Work out the finished part from the listing and answer in its coordinate system (mm). Face numbers are marked on the shaded views. A direction names the side the tool comes from. Round coordinates to 2 decimals unless told otherwise and drop trailing zeros. Order: outer loops, then holes, each group sorted by start corner. A loop starts at its lowest first (then second) coordinate and runs counter-clockwise, first axis right, second up. Notation, with made-up numbers: (13.25, 60) -> (41.25, 60) arc R27 cw to (41.25, 94) -> close; hole circle Ø9 at (3.25, 20). An arc over 180 degrees is marked (long way). Use a Markdown table: item, result. Add a question column.
Item 1: A cutting plane is placed at B-B, the plane z = 44. Determine the outline of the cut face in (x, y), plus the area to 3 significant figures.
Item 2: Flat-ended cylindrical pins translate along their axes: P1, Ø1, axis at y = -2.5, z = 32, coming from the -X side; P2, Ø8, axis at y = -5, z = 10, coming from the +X side; P3, Ø5, axis at y = 2, z = 54.5, coming from the -X side. Find the tip coordinate at first contact, or state that the pin passes through.
Item 3: A cutting plane is placed at A-A, the plane z = 13. Determine the outline of the cut face in (x, y), plus the area to 3 significant figures.
Item 4: Find the intervals of material crossed by L1, parallel to Y at x = 40, z = 55.75; L2, parallel to Z at x = 35, y = 5.5; L3, parallel to X at y = -1, z = 54, in increasing order. Write a range as [from, to].
Item 5: A cutting plane is placed at C-C, the plane x = -48.5. Determine the outline of the cut face in (y, z).
Item 6: A cutting plane is placed at D-D, the plane y = -12. Determine the outline of the cut face in (x, z), plus the area to 3 significant figures.
Item 7: For a pull along Z with two mould halves and no side action, classify the marked faces 1, 2, 3 and 4 as +Z half, -Z half, draft (parallel to the pull), parting line (faces both ways), or undercut.
Item 8: A tool of negligible diameter and unlimited length cuts with its end or side. For the marked faces 5, 6, 7 and 8, from which of +Z, -Z, +X, -X, +Y, -Y can it reach the whole face along a straight path? Write none if from no direction.
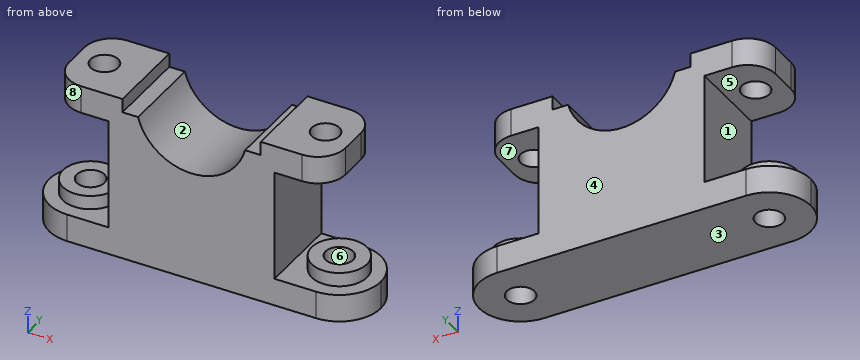
from build123d import *

# Parameters (mm, degrees)
F1_DEPTH         = 15
F2_R             = 10
F3_R             = 14.99999
F4_R             = 5
F5_DEPTH         = 10
F6_R             = 10
F7_DEPTH         = 5
F8_R             = 10
F9_DEPTH         = 5
F12_D            = 10
F12_DEPTH        = 15.001
F12_ON_F11_D     = 10
F12_ON_F11_DEPTH = 15.001


# Not quite as in the source:
# - a fillet or chamfer is up to 0.001 mm smaller than in the source, because OpenCascade refuses the exact size


with BuildPart() as f1:
    # F0 (on Front) → F1 (new body, symmetric)
    with BuildSketch(Plane.XZ):
        with BuildLine():
            Line((-60, 10), (-60, 0))
            Line((-60, 0), (60, 0))
            Line((60, 0), (60, 10))
            Line((60, 10), (30, 10))
            Line((30, 10), (30, 50))
            Line((30, 50), (50, 50))
            Line((50, 50), (50, 60))
            Line((50, 60), (25, 60))
            Line((25, 60), (25, 55))
            Line((25, 55), (19.364916731, 55))
            ThreePointArc((19.364916731, 55), (0, 40), (-19.364916731, 55))
            Line((-19.364916731, 55), (-25, 55))
            Line((-25, 55), (-25, 60))
            Line((-25, 60), (-50, 60))
            Line((-50, 60), (-50, 50))
            Line((-50, 50), (-30, 50))
            Line((-30, 50), (-30, 10))
            Line((-30, 10), (-60, 10))
        make_face()
    extrude(amount=F1_DEPTH, both=True)

    # F2
    f2_edges = [f1.edges().sort_by_distance(p)[0] for p in [
        (-50, -15, 55),
        (50, -15, 55),
        (50, 15, 55),
        (-50, 15, 55),
    ]]
    fillet(f2_edges, radius=F2_R)

    # F3 (radius 15 in the source; OpenCascade refuses exactly that, so slightly less here)
    f3_edges = [f1.edges().sort_by_distance(p)[0] for p in [
        (60, 15, 5),
        (-60, 15, 5),
        (-60, -15, 5),
        (60, -15, 5),
    ]]
    fillet(f3_edges, radius=F3_R)

    # F4 (on face) → F5 (cut, through all)
    with BuildSketch(Plane.XY.offset(60)):
        with Locations((40, 0)):
            Circle(F4_R)
        with Locations((-40, 0)):
            Circle(F4_R)
    extrude(amount=-F5_DEPTH, mode=Mode.SUBTRACT)

    # F6 (on face) → F7 (join)
    with BuildSketch(Plane.XY.offset(10)):
        with Locations((45, 0)):
            Circle(F6_R)
    extrude(amount=F7_DEPTH)

    # F8 (on face) → F9 (join)
    with BuildSketch(Plane.XY.offset(10)):
        with Locations((-45, 0)):
            Circle(F8_R)
    extrude(amount=F9_DEPTH)

    # F12 (through all, one way)
    with BuildSketch(Plane.XY.offset(15)):
        with Locations((-45, 0)):
            Circle(F12_D / 2)
    extrude(amount=-F12_DEPTH, mode=Mode.SUBTRACT)

    # F12 on F11 (through all, one way)
    with BuildSketch(Plane.XY.offset(15)):
        with Locations((45, 0)):
            Circle(F12_ON_F11_D / 2)
    extrude(amount=-F12_ON_F11_DEPTH, mode=Mode.SUBTRACT)


solid = f1.part
Reported:
| question | item | result |
|---|---|---|
| 1 | outline | (-30, -15) -> (-12, -15) -> (-12, 15) -> (-30, 15) -> close; (12, -15) -> (30, -15) -> (30, 15) -> (12, 15) -> close |
| 1 | area | 1,080 mm² |
| 2 | P1 | x = -30 |
| 2 | P2 | x = 59.97 |
| 2 | P3 | x = -50 |
| 3 | outline | circle Ø20 at (-45, 0); (-30, -15) -> (30, -15) -> (30, 15) -> (-30, 15) -> close; circle Ø20 at (45, 0); hole circle Ø10 at (-45, 0); hole circle Ø10 at (45, 0) |
| 3 | area | 2,270 mm² |
| 4 | L1 | [-15, -5], [5, 15] |
| 4 | L2 | [0, 10], [50, 60] |
| 4 | L3 | [-50, -44.9], [-35.1, -19.08], [19.08, 35.1], [44.9, 50] |
| 5 | outline | (-14.59, 0) -> (-3.57, 0) -> (-3.57, 15) -> (-9.37, 15) -> (-9.37, 10) -> (-14.59, 10) -> close; (-10.27, 50) -> (10.27, 50) -> (10.27, 60) -> (-10.27, 60) -> close; (3.57, 0) -> (14.59, 0) -> (14.59, 10) -> (9.37, 10) -> (9.37, 15) -> (3.57, 15) -> close |
| 6 | outline | (-54, 0) -> (54, 0) -> (54, 10) -> (30, 10) -> (30, 50) -> (47.14, 50) -> (47.14, 60) -> (25, 60) -> (25, 55) -> (19.36, 55) arc R20 cw to (-19.36, 55) -> (-25, 55) -> (-25, 60) -> (-47.14, 60) -> (-47.14, 50) -> (-30, 50) -> (-30, 10) -> (-54, 10) -> close |
| 6 | area | 3,740 mm² |
| 7 | face 1 | undercut |
| 7 | face 2 | +Z half |
| 7 | face 3 | -Z half |
| 7 | face 4 | draft |
| 8 | face 5 | -X, +Y, -Y |
| 8 | face 6 | -Z |
| 8 | face 7 | +X, +Y, -Y |
| 8 | face 8 | +Z, -X, -Y |
